Can you work these out from the model? Positions are in its coordinate system, mm. A direction names the side the tool comes from. Give positions to 0.01 mm unless a question says otherwise; leave off trailing zeros. Order: outer loops, then holes, each group sorted by start corner. A loop starts at its lowest first (then second) coordinate and runs counter-clockwise, first axis right, second up.
Item 1: I want a section at C-C, the plane x = 111.5. Write out the boundary of the cut face in (y, z).
Item 2: I want a section at D-D, the plane x = 93.5. Write out the boundary of the cut face in (y, z), then the cut area to 3 significant figures.
Item 3: I want a section at A-A, the plane z = -61.5. Write out the boundary of the cut face in (x, y), then the cut area to 3 significant figures.
Item 4: I'm going to push flat-ended pins straight in: pin 1 Ø10 at (y, z) = (15.5, -44.5) entering from -X; pin 2 Ø5 at (x, y) = (73, 17) entering from -Z. Where does each tip first touch, or does it pass through?
Item 5: If we mould it in two halves opening along Z, with no side actions, what happens to faces 1 (the flat face through (97, 15, -64.686)), 2 (the flat face through (128.5, 30, -53.7)), 3 (the cylindrical face through (65.3, 15.8, -53.4)), 4 (the flat face through (97, 16, -65.686))? For each: +Z half, -Z half, draft (parallel to the pull), parting line (faces both ways), or undercut.
Item 6: I want a section at B-B, the plane y = 5.5. Write out the boundary of the cut face in (x, z), then the cut area to 3 significant figures.
Item 7: If I drill on line 1 along Z through (x, y) = (100, 18); line 2 along Y through (x, z) = (73.5, -54.5); line 3 along X through (y, z) = (10.5, -52.25), over which ranges is the centre line in solid material (lowest first)?
Item 8: Which directions (+Z, -Z, +X, -X, +Y, -Y) give clear straight access to the entire face, cutting with the end or side of a thin tool? Please do faces 5 (the cylindrical face through (128.764, 30.986, -54.575)), 6 (the flat face through (85, 30, -54)), 7 (the cylindrical face through (128.296, 14.79, -53.928)).
```python
from build123d import *

# Parameters (mm, degrees)
BOSS_EXTRUDE1_DEPTH = 30
SKETCH3_R           = 11.5
BOSS_EXTRUDE2_DEPTH = 2


with BuildPart() as part:
    # Sketch2 → Boss-Extrude1 (new body)
    with BuildSketch(Plane(origin=(0, 0, 0), x_dir=(1, 0, 0), z_dir=(0, 1, 0))):
        with BuildLine():
            Line((77.29844251, 41.68564095), (117.29844251, 41.68564095))
            ThreePointArc((117.29844251, 41.68564095), (129.29844251, 53.68564095), (117.29844251, 65.68564095))
            Line((117.29844251, 65.68564095), (77.29844251, 65.68564095))
            ThreePointArc((77.29844251, 65.68564095), (65.29844251, 53.68564095), (77.29844251, 41.68564095))
        make_face()
        with BuildLine():
            Line((77.29844251, 64.68564095), (117.29844251, 64.68564095))
            ThreePointArc((117.29844251, 64.68564095), (128.29844251, 53.68564095), (117.29844251, 42.68564095))
            Line((117.29844251, 42.68564095), (77.29844251, 42.68564095))
            ThreePointArc((77.29844251, 42.68564095), (66.29844251, 53.68564095), (77.29844251, 64.68564095))
        make_face(mode=Mode.SUBTRACT)
    extrude(amount=BOSS_EXTRUDE1_DEPTH)

    # Sketch3 → Boss-Extrude2 (add)
    with BuildSketch(Plane(origin=(0, 30, 0), x_dir=(1, 0, 0), z_dir=(0, 1, 0))):
        with BuildLine():
            Line((77.29844251, 65.68564095), (117.29844251, 65.68564095))
            ThreePointArc((117.29844251, 65.68564095), (129.29844251, 53.68564095), (117.29844251, 41.68564095))
            Line((117.29844251, 41.68564095), (77.29844251, 41.68564095))
            ThreePointArc((77.29844251, 41.68564095), (65.29844251, 53.68564095), (77.29844251, 65.68564095))
        make_face()
        with Locations(Location((117.29844251, 53.68564095, 0), (0, 0, 106.957426294))):
            Circle(SKETCH3_R, mode=Mode.SUBTRACT)
    extrude(amount=BOSS_EXTRUDE2_DEPTH)


solid = part.part
```
Results list:
1. outline: (0, -65.69) - (32, -65.69) - (32, -63.62) - (30, -63.62) - (30, -64.69) - (0, -64.69) - close; (0, -42.69) - (30, -42.69) - (30, -43.75) - (32, -43.75) - (32, -41.69) - (0, -41.69) - close
2. outline: (0, -65.69) - (32, -65.69) - (32, -41.69) - (0, -41.69) - (0, -42.69) - (30, -42.69) - (30, -64.69) - (0, -64.69) - close
2. area: 108 mm2
3. outline: (68.19, 0) - (69.56, 0) - (69.56, 30) - (108.86, 30) - (108.86, 32) - (68.19, 32) - close; (125.04, 0) - (126.41, 0) - (126.41, 32) - (125.74, 32) - (125.74, 30) - (125.04, 30) - close
3. area: 165 mm2
4. pin 1: stops at x = 66.05
4. pin 2: stops at z = -65.55
5. face 1: undercut
5. face 2: undercut
5. face 3: parting line
5. face 4: -Z half
6. outline: (77.3, -65.69) - (117.3, -65.69) arc R12 ccw to (117.3, -41.69) - (77.3, -41.69) arc R12 ccw to start; hole (77.3, -64.69) - (117.3, -64.69) arc R11 ccw to (117.3, -42.69) - (77.3, -42.69) arc R11 ccw to start
6. area: 152 mm2
7. line 1: z = -65.69 to -64.69, -42.69 to -41.69
7. line 2: y = 30 to 32
7. line 3: x = 65.38 to 66.39, 128.2 to 129.21
8. face 5: +Y
8. face 6: -Y
8. face 7: +Y, -Y
